from build123d import *

# Parameters (mm, degrees)
SKETCH1_W           = 94.8
SKETCH1_H           = 69.85
SKETCH1_R           = 2.25
SKETCH1_R_2         = 1.45
SKETCH1_R_3         = 3.25755
SKETCH1_R_4         = 19.5
BOSS_EXTRUDE1_DEPTH = 6.35
CUT_EXTRUDE2_DEPTH  = 3


with BuildPart() as part:
    # Sketch1 → Boss-Extrude1 (new body)
    with BuildSketch(Plane(origin=(0, 0, 0), x_dir=(1, 0, 0), z_dir=(0, 1, 0))):
        Rectangle(SKETCH1_W, SKETCH1_H)
        with Locations((-17.138337536, -28.111820997)):
            Circle(SKETCH1_R, mode=Mode.SUBTRACT)
        with Locations((20.56810334, 19.875)):
            Circle(SKETCH1_R_2, mode=Mode.SUBTRACT)
        with Locations((-20.56810334, 19.875)):
            Circle(SKETCH1_R_2, mode=Mode.SUBTRACT)
        with Locations((0, -15.75)):
            Circle(SKETCH1_R_2, mode=Mode.SUBTRACT)
        with Locations((34.7, 3.175)):
            Circle(SKETCH1_R_3, mode=Mode.SUBTRACT)
        with Locations((-34.7, 3.175)):
            Circle(SKETCH1_R_3, mode=Mode.SUBTRACT)
        with Locations((0, 8)):
            Circle(SKETCH1_R_4, mode=Mode.SUBTRACT)
        with Locations((-11.164910261, -22.79033938)):
            Circle(SKETCH1_R, mode=Mode.SUBTRACT)
        with Locations((-34.7, -22.225)):
            Circle(SKETCH1_R_3, mode=Mode.SUBTRACT)
        with Locations((34.7, -22.225)):
            Circle(SKETCH1_R_3, mode=Mode.SUBTRACT)
    extrude(amount=BOSS_EXTRUDE1_DEPTH)

    # Sketch4 → Cut-Extrude2 (cut)
    with BuildSketch(Plane.XZ):
        with BuildLine():
            Line((-14.145004126, 31.471873838), (-8.171576852, 26.150392222))
            ThreePointArc((-8.171576852, 26.150392222), (-7.804857419, 19.797005971), (-14.15824367, 19.430286538))
            Line((-14.15824367, 19.430286538), (-20.131670945, 24.751768155))
            ThreePointArc((-20.131670945, 24.751768155), (-20.498390378, 31.105154406), (-14.145004126, 31.471873838))
        make_face()
    extrude(amount=-CUT_EXTRUDE2_DEPTH, mode=Mode.SUBTRACT)


solid = part.part
Could you check a few things on this model? Use its own coordinates, in mm. A direction names the side the tool comes from. Give positions to 0.01 mm unless a question says otherwise; leave off trailing zeros. Order: outer loops, then holes, each group sorted by start corner. A loop starts at its lowest first (then second) coordinate and runs counter-clockwise, first axis right, second up. Notation, with made-up numbers: (83.25, 37.5) -> (108.25, 37.5) arc R3 cw to (108.25, 41.5) -> close; hole circle Ø4 at (-15.75, 5). An arc over 180 degrees is marked (long way). Return JSON: item names as keys, results as strings.
1. On a 3-axis mill with a long thin cutter (end or side, diameter ignored), from which of +Z, -Z, +X, -X, +Y, -Y can I reach the whole of each face in a straight line? I mean faces 1 (the flat face through (10, 0, 15)), 2 (the flat face through (-11.2, 1.48, 28.85)). Say none if no direction works.
Answer list:
{"face 1": "+Z, -Z, +X, -X, -Y", "face 2": "-Y"}
2. Imagine slicing it at A-A on x = 0. List the corners of the cut face in (y, z) for me (3 decimals).
Answer list:
{"outline": "(0, -34.925) -> (6.35, -34.925) -> (6.35, -27.5) -> (0, -27.5) -> close; (0, 11.5) -> (6.35, 11.5) -> (6.35, 14.3) -> (0, 14.3) -> close; (0, 17.2) -> (6.35, 17.2) -> (6.35, 34.925) -> (0, 34.925) -> close"}
3. Imagine slicing it at B-B on z = -8. List the corners of the cut face in (x, y) for me, then the cut area to 3 significant figures.
Answer list:
{"outline": "(-47.4, 0) -> (-19.5, 0) -> (-19.5, 6.35) -> (-47.4, 6.35) -> close; (19.5, 0) -> (47.4, 0) -> (47.4, 6.35) -> (19.5, 6.35) -> close", "area": "354 mm2"}
4. Imagine slicing it at D-D on x = -34.7. List the corners of the cut face in (y, z) for me (3 decimals).
Answer list:
{"outline": "(0, -34.925) -> (6.35, -34.925) -> (6.35, -6.433) -> (0, -6.433) -> close; (0, 0.083) -> (6.35, 0.083) -> (6.35, 18.967) -> (0, 18.967) -> close; (0, 25.483) -> (6.35, 25.483) -> (6.35, 34.925) -> (0, 34.925) -> close"}
5. Imagine slicing it at C-C on z = 15.75. List the corners of the cut face in (x, y) for me, then the cut area to 3 significant figures.
Answer list:
{"outline": "(-47.4, 0) -> (-1.45, 0) -> (-1.45, 6.35) -> (-47.4, 6.35) -> close; (1.45, 0) -> (47.4, 0) -> (47.4, 6.35) -> (1.45, 6.35) -> close", "area": "584 mm2"}
6. Thinking about a two-plate mould opening in Z: for faces 3 (the flat face through (-47.4, 3, 0)), 4 (the cylindrical face through (-37.954, 3.131, -3.318)), 5 (the flat face through (-1, 3, 34.925)), which applies, pulls with the +Z half, pulls with the -Z half, needs draft (parallel to the pull), parting line crosses it, or undercut?
Answer list:
{"face 3": "needs draft", "face 4": "undercut", "face 5": "pulls with the +Z half"}
7. For pin 1 Ø6 at (x, z) = (34.7, 22.225) entering from -Y; pin 2 Ø5 at (x, z) = (-17.14, 28.11) entering from -Y, each with a flat end and sliding along its axis, tell me the tip position at first contact or that it passes through.
Answer list:
{"pin 1": "passes through", "pin 2": "stops at y = 3"}
8. I need wall thicknesses on line 1 (Z direction, x = 0, y = 3.75) (3 decimals); line 2 (Z direction, x = -34.7, y = 2) (3 decimals); line 3 (X direction, y = 5.5, z = -8). Which ranges of each line are inside material? Lowest first, please. Write a range as from..to.
Answer list:
{"line 1": "z = -34.925..-27.5, 11.5..14.3, 17.2..34.925", "line 2": "z = -34.925..-6.433, 0.083..18.967, 25.483..34.925", "line 3": "x = -47.4..-19.5, 19.5..47.4"}
